For this review, take the finished solid that the model builds, in its own axes (mm). Face numbers are marked on the shaded views. Coordinates: 2 decimals unless noted, no trailing zeros. Write each loop counter-clockwise with the first axis right and the second up, starting at its lowest first coordinate (ties: lowest second). Pieces come first, ordered by that corner, then holes. Notation, with made-up numbers: (-22.5, -14) -> (0.5, -14) arc R14 ccw to (0.5, 4) -> close; hole circle Ø5 at (18, -35). An arc over 180 degrees is marked (long way). Put each result on its own line as item: value. Start each with the question number.
Item 1: Consider section A-A on x = -19.5. Give the boundary of the cut face in (y, z).
Item 2: Consider section B-B on z = 2.15. Give the number of separate pieces and of enclosed holes in the cut face, and give its area (3 significant figures).
Item 3: Consider section C-C on y = 30.5. Give the boundary of the cut face in (x, z).
Item 4: To check wall thickness, follow L1, parallel to X at y = -3.5, z = 2; L2, parallel to X at y = 5.5, z = 0.2; L3, parallel to Y at x = -9, z = 1.05. State the ranges of each line that lie inside material, in increasing order.
Item 5: Insertion check: P1, Ø1, axis at y = 28.5, z = 2.5, coming from the -X side. The pin has a flat end and moves straight along its axis. Give the tip position at first contact, or say it passes through.
Item 6: The part is to be moulded in two halves that separate along Y. For the marked faces 1, 2 and 3, say which applies: +Y half, -Y half, draft (parallel to the pull), parting line (faces both ways), or undercut.
```python
from build123d import *

# Parameters (mm, degrees)
SKETCH1_R           = 6
SKETCH1_R_2         = 2.15
BOSS_EXTRUDE3_DEPTH = 2.8
FILLET2_R           = 0.5


with BuildPart() as part:
    # Sketch1 → Boss-Extrude3 (new body)
    with BuildSketch(Plane.XY):
        with BuildLine():
            Line((-6.914903584, -6.003890728), (-32.597767901, 37.912867577))
            Line((-32.597767901, 37.912867577), (10.012592639, 3.48020667))
            add(Edge.make_bspline(
                [(10.012592639, 3.48020667), (13.976241168, 1.192727745), (14.014521415, -3.518986682), (16.534972158, -6.795729316)],
                knots=[0, 0, 0, 0, 1, 1, 1, 1], degree=3))
            add(Edge.make_bspline(
                [(-6.914903584, -6.003890728), (-3.45265208, -9.610347217), (5.034074198, -6.462522657), (13.416090218, -10.783276778), (16.534972158, -6.795729316)],
                knots=[0, 0, 0, 0, 0.517120054, 1, 1, 1, 1], degree=3))
        make_face()
        Circle(SKETCH1_R, mode=Mode.SUBTRACT)
        with Locations((-7.406949835, 6.718414556)):
            Circle(SKETCH1_R_2, mode=Mode.SUBTRACT)
        with Locations((9.329230051, -3.600759177)):
            Circle(SKETCH1_R_2, mode=Mode.SUBTRACT)
    extrude(amount=BOSS_EXTRUDE3_DEPTH)

    # Fillet2
    fillet2_edges = [part.edges().sort_by_distance(p)[0] for p in [
        (16.534972158, -6.795729316, 1.4),
    ]]
    fillet(fillet2_edges, radius=FILLET2_R)


solid = part.part
```
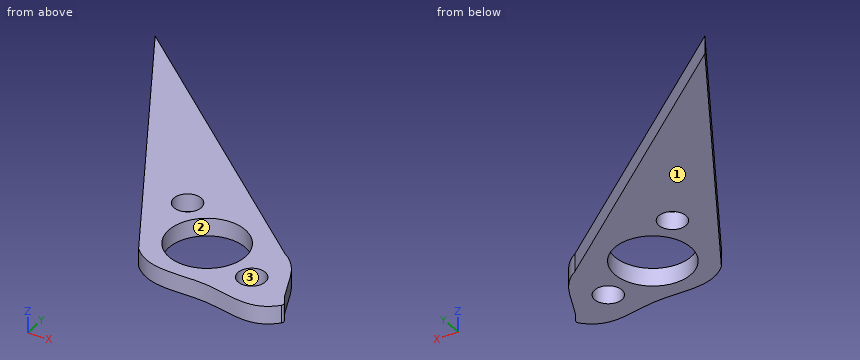
Return value:
1. outline: (15.52, 0) -> (27.33, 0) -> (27.33, 2.8) -> (15.52, 2.8) -> close
2. separate pieces: 1
2. enclosed holes: 3
2. area: 520 mm^2
3. outline: (-28.26, 0) -> (-23.42, 0) -> (-23.42, 2.8) -> (-28.26, 2.8) -> close
4. L1: -8.38 to -4.87, 4.87 to 7.18, 11.48 to 14.74
4. L2: -13.64 to -9.18, -5.64 to -2.4, 2.4 to 7.51
4. L3: -2.44 to 5.27, 8.16 to 18.84
5. P1: x = -27.39
6. face 1: draft
6. face 2: undercut
6. face 3: undercut
